Check sheet for the modelled part. Datum: model origin and axes. Units: mm. A direction names the side the tool comes from. Coordinates: 2 decimals unless noted, no trailing zeros. Loops run counter-clockwise (first coordinate to the right, second up) from the corner with the lowest first, then second, coordinate; pieces in that order, holes last. Notation, with made-up numbers: (63.25, 4.5) - (115.25, 4.5) arc R19 ccw to (115.25, 36.5) - close; hole circle Ø9 at (53.5, 79.25). An arc over 180 degrees is marked (long way). Use a Markdown table: item, result. Add a question column.
1) Tool access check on faces 4 (the flat face through (-48, -92.5, -17)), 5 (the cylindrical face through (7.587, 70.315, 34.168)), 6 (the cylindrical face through (-47.69, -92.25, -15.02)). Record the directions out of +Z, -Z, +X, -X, +Y, -Y that give a thin tool (end or side, any length) a straight path to the whole face; none if there is none.
2) Sectioned sample at B-B, the plane x = 0. Enter the section's corners in (y, z).
3) Thickness scan on line 1 (Z direction, x = 0, y = -92); line 2 (Z direction, x = 0, y = 54.5); line 3 (Y direction, x = -56.5, z = 21). Record the ranges inside material, lowest first.
4) Sectioned sample at D-D, the plane y = -12. Enter the section's corners in (x, z), then the cut area to 3 significant figures.
5) Draft check along X on faces 1 (the flat face through (-57, -72.5, 0)), 2 (the conical face through (8.01, -1.42, 36.06)), 3 (the conical face through (25.48, -30.47, 19.54)). Enter one of: pulls with the +X half, pulls with the -X half, needs draft (parallel to the pull), parting line crosses it, or undercut.
6) Go/stop test with flat-tipped pins: P1, Ø2, axis at x = -19.5, y = -60, coming from the +Z side; P2, Ø1, axis at x = -37.5, z = -38, coming from the +Y side; P3, Ø4, axis at y = 67, z = -12, coming from the -X side. Record where each tip stops, or that it passes through.
7) Sectioned sample at C-C, the plane y = 62. Enter the section's corners in (x, z), then the cut area to 3 significant figures.
8) Sectioned sample at A-A, the plane z = 0. Enter the section's corners in (x, y).
from build123d import *


with BuildPart() as part:
    # Sketch3 → Revolve1 (revolve)
    with BuildSketch(Plane.XY, mode=Mode.PRIVATE) as revolve1_sk:
        with BuildLine():
            Line((25, 92.5), (25, 8.21170714))
            Line((25, 8.21170714), (42.956663453, -89.5))
            Line((42.956663453, -89.5), (47.5, -89.5))
            ThreePointArc((47.5, -89.5), (49.267766953, -90.232233047), (50, -92))
            Line((50, -92), (50, -92.5))
            Line((50, -92.5), (70, -92.5))
            Line((70, -92.5), (70, -72.5))
            Line((70, -72.5), (56.663791728, -72.5))
            ThreePointArc((56.663791728, -72.5), (51.543620306, -70.646856482), (48.795552004, -65.945961153))
            Line((48.795552004, -65.945961153), (29.610902689, 38.447866821))
            ThreePointArc((29.610902689, 38.447866821), (30.60510735, 43.986216269), (35, 47.5))
            Line((35, 47.5), (35, 92.5))
            Line((35, 92.5), (25, 92.5))
        make_face()
    revolve(revolve1_sk.sketch.rotate(Axis((0, 92.5, 0), (0, -1, 0)), 180), axis=Axis((0, 92.5, 0), (0, -1, 0)))


solid = part.part
Solved:
| question | item | result |
|---|---|---|
| 1 | face 4 | +Z, -Z, +X, -X, -Y |
| 1 | face 5 | +Y |
| 1 | face 6 | -Y |
| 2 | outline | (-92.5, -70) - (-72.5, -70) - (-72.5, -56.66) arc R8 cw to (-65.95, -48.8) - (38.45, -29.61) arc R8 cw to (47.5, -35) - (92.5, -35) - (92.5, -25) - (8.21, -25) - (-89.5, -42.96) - (-89.5, -47.5) arc R2.5 cw to (-92, -50) - (-92.5, -50) - close; (-92.5, 50) - (-92, 50) arc R2.5 cw to (-89.5, 47.5) - (-89.5, 42.96) - (8.21, 25) - (92.5, 25) - (92.5, 35) - (47.5, 35) arc R8 cw to (38.45, 29.61) - (-65.95, 48.8) arc R8 cw to (-72.5, 56.66) - (-72.5, 70) - (-92.5, 70) - close |
| 3 | line 1 | z = -70 to -50, 50 to 70 |
| 3 | line 2 | z = -35 to -25, 25 to 35 |
| 3 | line 3 | y = -92.5 to -72.5 |
| 4 | outline | circle Ø77.76 at (0, 0); hole circle Ø57.43 at (0, 0) |
| 4 | area | 2,160 mm2 |
| 5 | face 1 | needs draft |
| 5 | face 2 | parting line crosses it |
| 5 | face 3 | undercut |
| 6 | P1 | stops at z = 44.01 |
| 6 | P2 | stops at y = -71.55 |
| 6 | P3 | stops at x = -33.54 |
| 7 | outline | circle Ø70 at (0, 0); hole circle Ø50 at (0, 0) |
| 7 | area | 1,880 mm2 |
| 8 | outline | (-70, -92.5) - (-50, -92.5) - (-50, -92) arc R2.5 cw to (-47.5, -89.5) - (-42.96, -89.5) - (-25, 8.21) - (-25, 92.5) - (-35, 92.5) - (-35, 47.5) arc R8 cw to (-29.61, 38.45) - (-48.8, -65.95) arc R8 cw to (-56.66, -72.5) - (-70, -72.5) - close; (25, 8.21) - (42.96, -89.5) - (47.5, -89.5) arc R2.5 cw to (50, -92) - (50, -92.5) - (70, -92.5) - (70, -72.5) - (56.66, -72.5) arc R8 cw to (48.8, -65.95) - (29.61, 38.45) arc R8 cw to (35, 47.5) - (35, 92.5) - (25, 92.5) - close |
